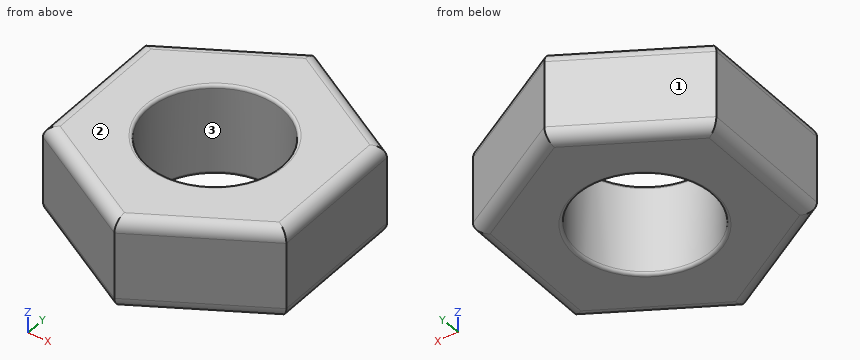
from build123d import *

# Parameters (mm, degrees)
SKETCH_1_R      = 11
EXTRUDE_1_DEPTH = 15
FILLET_1_R      = 2
FILLET_2_R      = 0.5


with BuildPart() as part:
    # 草图1 → 凸台-拉伸1 (new body)
    with BuildSketch(Plane.XY):
        Polygon((0, -23.094010768), (20, -11.547005384), (20, 11.547005384), (0, 23.094010768), (-20, 11.547005384), (-20, -11.547005384), align=None)
        Circle(SKETCH_1_R, mode=Mode.SUBTRACT)
    extrude(amount=EXTRUDE_1_DEPTH)

    # 圆角1
    fillet_1_edges = [part.edges().sort_by_distance(p)[0] for p in [
        (20, 0, 15),
        (10, 17.320508076, 15),
        (-10, 17.320508076, 15),
        (-20, 0, 15),
        (-10, -17.320508076, 15),
        (-20, 0, 0),
        (-10, 17.320508076, 0),
        (10, 17.320508076, 0),
        (10, -17.320508076, 15),
        (20, 0, 0),
        (10, -17.320508076, 0),
        (-10, -17.320508076, 0),
    ]]
    fillet(fillet_1_edges, radius=FILLET_1_R)

    # 圆角2
    fillet_2_edges = [part.edges().sort_by_distance(p)[0] for p in [
        (-11, 0, 0),
        (-11, 0, 15),
    ]]
    fillet(fillet_2_edges, radius=FILLET_2_R)


solid = part.part
Check sheet for the modelled part. Datum: model origin and axes. Units: mm. Face numbers are marked on the shaded views. Give positions to 0.01 mm unless a question says otherwise; leave off trailing zeros. Order: outer loops, then holes, each group sorted by start corner. A loop starts at its lowest first (then second) coordinate and runs counter-clockwise, first axis right, second up. Notation, with made-up numbers: (59.25, -9) - (116.25, -9) arc R14 ccw to (116.25, 14) - close; hole circle Ø1 at (7, -39). An arc over 180 degrees is marked (long way). Answer as CSV lines item,"result".
1. Section check B-B (y = 0). Record the boundary of the cut face in (x, z).
Result sheet:
outline,"(-20, 2) arc R2 ccw to (-18, 0) - (-11.5, 0) arc R0.5 ccw to (-11, 0.5) - (-11, 14.5) arc R0.5 ccw to (-11.5, 15) - (-18, 15) arc R2 ccw to (-20, 13) - close; (11, 0.5) arc R0.5 ccw to (11.5, 0) - (18, 0) arc R2 ccw to (20, 2) - (20, 13) arc R2 ccw to (18, 15) - (11.5, 15) arc R0.5 ccw to (11, 14.5) - close"
2. Go/stop test with flat-tipped pins: P1, Ø4, axis at x = 9.5, z = 12, coming from the -Y side; P2, Ø10, axis at x = 10.5, y = -0.5, coming from the -Z side; P3, Ø5, axis at x = 6, z = 12.5, coming from the +Y side; P4, Ø1, axis at x = 14.5, y = 14.5, coming from the +Z side. Record where each tip stops, or that it passes through.
Result sheet:
P1,"y = -18.76"
P2,"z = 0"
P3,"y = 21.07"
P4,"z = 14.51"
3. Mould release check, pull along Y, two halves, no side actions. Record for the marked faces 1, 2 and 3: released by +Y, released by -Y, zero draft, split by the parting line, or undercut.
Result sheet:
face 1,"released by +Y"
face 2,"zero draft"
face 3,"undercut"
4. Section check A-A (z = 3). Record the boundary of the cut face in (x, y).
Result sheet:
outline,"(-20, -11.55) - (0, -23.09) - (20, -11.55) - (20, 11.55) - (0, 23.09) - (-20, 11.55) - close; hole circle Ø22 at (0, 0)"
5. Scan lines: probe 1 along X at (y, z) = (-4.5, 0.75); probe 2 along X at (y, z) = (-9.5, 1.25); probe 3 along Y at (x, z) = (0, 4.75). Record each from-to range of solid material in increasing order. Write a range as from..to.
Result sheet:
probe 1,"-19.56..-10.04, 10.04..19.56"
probe 2,"-19.85..-5.55, 5.55..19.85"
probe 3,"-23.09..-11, 11..23.09"
